Verification items for the finished model (mm, model axes). A direction names the side the tool comes from. Coordinates: 2 decimals unless noted, no trailing zeros. Write each loop counter-clockwise with the first axis right and the second up, starting at its lowest first coordinate (ties: lowest second). Pieces come first, ordered by that corner, then holes. Notation, with made-up numbers: M 66,-17 L 98,-17 A31 cw 98,20 Z; hole C 72,13.25 d2. An arc over 180 degrees is marked long. Answer in a Markdown table with one row per item.
from build123d import *

# Parameters (mm, degrees)
SKETCH1_R           = 0.6985
SKETCH1_R_2         = 0.7874
BOSS_EXTRUDE1_DEPTH = 0.508
SKETCH3_R           = 2.794
SKETCH4_R           = 2.147566379
SKETCH5_R           = 1.067023976
SKETCH6_R           = 0.7874
CUT_EXTRUDE1_START  = -0.508
SKETCH7_R           = 0.7874
CUT_EXTRUDE1_DEPTH  = 0.508
BOSS_EXTRUDE2_DEPTH = 0.889
BOSS_EXTRUDE3_DEPTH = 0.889
FILLET1_R           = 0.508


with BuildPart() as part:
    # Sketch1 → Boss-Extrude1 (new body)
    with BuildSketch(Plane.XY):
        with BuildLine():
            Line((0.889, 0), (9.906, 0))
            ThreePointArc((9.906, 0), (10.534617928, 0.260382072), (10.795, 0.889))
            Line((10.795, 0.889), (10.795, 4.405000935))
            Line((10.795, 4.405000935), (9.871541288, 4.405000935))
            Line((9.871541288, 4.405000935), (9.871541288, 7.2898))
            Line((9.871541288, 7.2898), (10.795, 7.2898))
            Line((10.795, 7.2898), (10.795, 10.414))
            ThreePointArc((10.795, 10.414), (10.534617928, 11.042617928), (9.906, 11.303))
            Line((9.906, 11.303), (0.889, 11.303))
            ThreePointArc((0.889, 11.303), (0.260382072, 11.042617928), (0, 10.414))
            Line((0, 10.414), (0, 7.2898))
            Line((0, 7.2898), (0.923458712, 7.2898))
            Line((0.923458712, 7.2898), (0.923458712, 4.405000935))
            Line((0.923458712, 4.405000935), (0, 4.405000935))
            Line((0, 4.405000935), (0, 0.889))
            ThreePointArc((0, 0.889), (0.260382072, 0.260382072), (0.889, 0))
        make_face()
        with Locations((5.3975, 10.033)):
            Circle(SKETCH1_R, mode=Mode.SUBTRACT)
        with Locations((5.3975, 1.5494)):
            Circle(SKETCH1_R_2, mode=Mode.SUBTRACT)
    extrude(amount=BOSS_EXTRUDE1_DEPTH)

    # Sketch3 → Loft1 section 0
    with BuildSketch(Plane.XY.offset(0.508)):
        with Locations((5.3975, 5.7912)):
            Circle(SKETCH3_R)
    # Sketch4 → Loft1 section 1
    with BuildSketch(Plane.XY.offset(1.9558)):
        with Locations((5.3975, 5.7912)):
            Circle(SKETCH4_R)
    loft()

    # Sketch5 → Loft2 section 0
    with BuildSketch(Plane.XY.offset(0.508)):
        with Locations((5.3975, 1.5494)):
            Circle(SKETCH5_R)
    # Sketch6 → Loft2 section 1
    with BuildSketch(Plane.XY.offset(1.016)):
        with Locations((5.3975, 1.5494)):
            Circle(SKETCH6_R)
    loft()

    # Sketch7 → Cut-Extrude1 (cut)
    with BuildSketch(Plane.XY.offset(1.016).offset(CUT_EXTRUDE1_START)):
        with Locations((5.3975, 1.5494)):
            Circle(SKETCH7_R)
    extrude(amount=CUT_EXTRUDE1_DEPTH, mode=Mode.SUBTRACT)

    # Sketch9 → Boss-Extrude2 (add)
    with BuildSketch(Plane.ZY):
        Polygon((0, 4.405000935), (0.956058861, 7.4), (1.44, 7.245517076), (0.508, 4.405000935), align=None)
    extrude(amount=-BOSS_EXTRUDE2_DEPTH)

    # Sketch10 → Boss-Extrude3 (add)
    with BuildSketch(Plane(origin=(10.795, 0, 0), x_dir=(0, 0, -1), z_dir=(1, 0, 0))):
        Polygon((-1.44, 7.245517076), (-0.508, 4.405000935), (0, 4.405000935), (-0.956058861, 7.4), align=None)
    extrude(amount=-BOSS_EXTRUDE3_DEPTH)

    # Fillet1
    # the kernel refuses this fillet: 0.508 mm, written as the material it adds along each edge
    with BuildSketch(Plane(origin=(10.795, 4.405000935, 0.508), x_dir=(0, -1, 0), z_dir=(-1, 0, 0)), Plane(origin=(0.889, 4.405000935, 0.508), x_dir=(0, -1, 0), z_dir=(-1, 0, 0))) as fillet1_piece_1:
        with BuildLine():
            CenterArc((FILLET1_R * 0.159862126559, FILLET1_R), FILLET1_R, 251.83485126, 18.16514874)
            Line((-FILLET1_R * 0.151894895434, FILLET1_R * 0.0498381405053), (0, 0))
            Line((0, 0), (FILLET1_R * 0.159862126559, 0))
        make_face()
    extrude(amount=0.889)
    with BuildSketch(Plane(origin=(5.3975, 5.7912, 0.508), x_dir=(1, 0, 0), z_dir=(0, -1, 0))) as fillet1_piece_2:
        with BuildLine():
            CenterArc((2.794 + FILLET1_R * 0.648657698793, FILLET1_R), FILLET1_R, 204.060462248, 65.939537752)
            Line((2.794 - FILLET1_R * 0.264458035208, FILLET1_R * 0.592299550749), (2.794, 0))
            Line((2.794, 0), (2.794 + FILLET1_R * 0.648657698793, 0))
        make_face()
    revolve(axis=Axis((5.3975, 5.7912, 0.508), (0, 0, 1)))
    with BuildSketch(Plane(origin=(5.3975, 1.5494, 0.508), x_dir=(1, 0, 0), z_dir=(0, -1, 0))) as fillet1_piece_3:
        with BuildLine():
            CenterArc((1.067023976 + FILLET1_R * 0.591042865148, FILLET1_R), FILLET1_R, 208.830184855, 61.169815145)
            Line((1.067023976 - FILLET1_R * 0.285009893371, FILLET1_R * 0.517784732415), (1.067023976, 0))
            Line((1.067023976, 0), (1.067023976 + FILLET1_R * 0.591042865148, 0))
        make_face()
    revolve(axis=Axis((5.3975, 1.5494, 0.508), (0, 0, 1)))
    # the kernel refuses this fillet: 0.508 mm, written as the material it takes off along each edge
    with BuildSketch(Plane(origin=(5.3975, 5.7912, 1.9558), x_dir=(1, 0, 0), z_dir=(0, -1, 0))) as fillet1_2_piece_1:
        with BuildLine():
            CenterArc((2.147566379 - FILLET1_R * 0.648657698793, -FILLET1_R), FILLET1_R, 24.060462248, 65.939537752)
            Line((2.147566379 - FILLET1_R * 0.648657698793, 0), (2.147566379, 0))
            Line((2.147566379, 0), (2.147566379 + FILLET1_R * 0.264458035208, -FILLET1_R * 0.592299550749))
        make_face()
    revolve(axis=Axis((5.3975, 5.7912, 1.9558), (0, 0, 1)), mode=Mode.SUBTRACT)


solid = part.part
1) Sectioned sample at A-A (y = 9.5). Record the cut outline in (x, z) (3 decimals), then the cut area to 3 significant figures.
Response values:
| item | result |
|---|---|
| outline | M 0,0 L 4.946,0 L 4.946,0.508 L 0,0.508 Z; M 5.849,0 L 10.795,0 L 10.795,0.508 L 5.849,0.508 Z |
| area | 5.03 mm² |
2) Thickness scan on L1, parallel to Y at x = 5, z = 0.2; L2, parallel to Z at x = 9, y = 1.25; L3, parallel to Y at x = 5, z = 1.85. Record the ranges inside material, lowest first. Write a range as [from, to].
Response values:
| item | result |
|---|---|
| L1 | y = [0, 0.87], [2.23, 9.46], [10.61, 11.3] |
| L2 | z = [0, 0.51] |
| L3 | y = [3.7, 7.88] |
3) Tool access check on faces 1 (the face through (10.4, 5.9, 1)), 2 (the face through (5, 6, 1.956)). Record the directions out of +Z, -Z, +X, -X, +Y, -Y that give a thin tool (end or side, any length) a straight path to the whole face; none if there is none.
Response values:
| item | result |
|---|---|
| face 1 | +Z, +X, -Y |
| face 2 | +Z, +X, -X, +Y, -Y |
4) Release check for a two-part mould opening along Y. For faces 3 (the face through (6.064, 10.243, 0.25)), 4 (the face through (5, 6, 0)), 5 (the face through (0.4, 5.9, 1)), 6 (the face through (0.44, 5.88, 0.47)) record: +Y half, -Y half, draft (parallel to the pull), parting line (faces both ways), or undercut.
Response values:
| item | result |
|---|---|
| face 3 | undercut |
| face 4 | draft |
| face 5 | -Y half |
| face 6 | undercut |
5) Sectioned sample at C-C (x = 2). Record the cut outline in (y, z), then the cut area to 3 significant figures.
Response values:
| item | result |
|---|---|
| outline | M 0,0 L 11.3,0 L 11.3,0.51 L 0,0.51 Z |
| area | 5.74 mm² |
6) Sectioned sample at B-B (z = 0.2). Give the number of separate pieces and of enclosed holes in the cut face, then the cut area to 3 significant figures.
Response values:
| item | result |
|---|---|
| separate pieces | 1 |
| enclosed holes | 2 |
| area | 114 mm² |
7) Depth check by flat-ended pin: pin 1 (0.8 mm diameter, centred on x = 5.4, y = 10.03, fed in from +Z); pin 2 (1.8 mm diameter, centred on x = 5.4, y = 1.55, fed in from +Z). Enter the tip coordinate at first touch or a pass-through.
Response values:
| item | result |
|---|---|
| pin 1 | passes through |
| pin 2 | stops at z = 1.02 |
